Here's the drawing with two shaded views (mm, measured from the low corner). I have some questions. Coordinates: 2 decimals unless noted, no trailing zeros. Write each loop counter-clockwise with the first axis right and the second up, starting at its lowest first coordinate (ties: lowest second). Pieces come first, ordered by that corner, then holes.
Item 1: If we section it at D-D (x = 3.3): Please give me the cut outline in (y, z), then the cut area to 3 significant figures.
Item 2: If I drill on line 1 (Y direction, x = 3.15, z = 10); line 2 (Z direction, x = 3.05, y = 15); line 3 (Y direction, x = 2.6, z = 65), over which ranges is the centre line in solid material (lowest first)?
Item 3: If we section it at B-B (y = 25): Please give me the cut outline in (x, z), then the cut area to 3 significant figures.
Item 4: If we section it at C-C (z = 65): Please give me the cut outline in (x, y).
Item 5: If we section it at A-A (z = 10): Please give me the cut outline in (x, y), then the cut area to 3 significant figures.
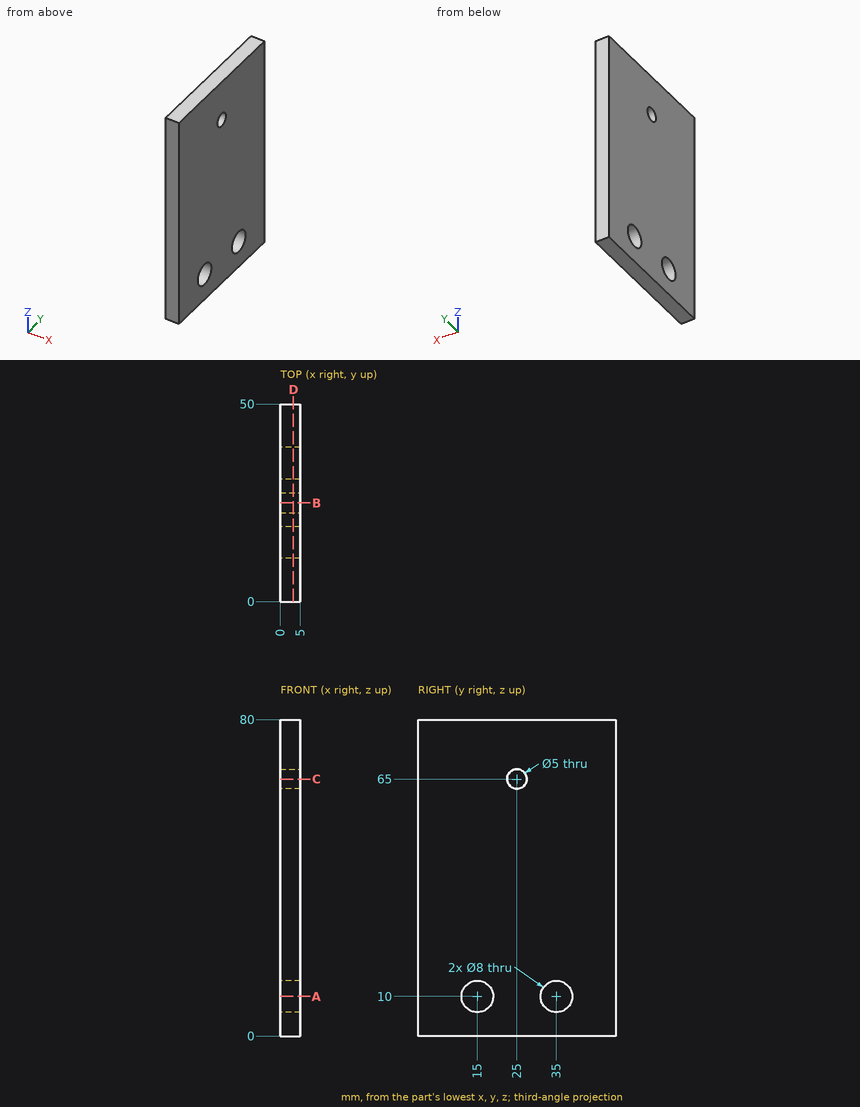
Answer list:
1. outline: (0, 0) - (50, 0) - (50, 80) - (0, 80) - close; hole circle Ø8 at (15, 10); hole circle Ø5 at (25, 65); hole circle Ø8 at (35, 10)
1. area: 3,880 mm2
2. line 1: y = 0 to 11, 19 to 31, 39 to 50
2. line 2: z = 0 to 6, 14 to 80
2. line 3: y = 0 to 22.5, 27.5 to 50
3. outline: (0, 0) - (5, 0) - (5, 62.5) - (0, 62.5) - close; (0, 67.5) - (5, 67.5) - (5, 80) - (0, 80) - close
3. area: 375 mm2
4. outline: (0, 0) - (5, 0) - (5, 22.5) - (0, 22.5) - close; (0, 27.5) - (5, 27.5) - (5, 50) - (0, 50) - close
5. outline: (0, 0) - (5, 0) - (5, 11) - (0, 11) - close; (0, 19) - (5, 19) - (5, 31) - (0, 31) - close; (0, 39) - (5, 39) - (5, 50) - (0, 50) - close
5. area: 170 mm2
